Solid Edge part; units mm, degrees
sketch "Sketch1" plane through (0, 0, 0) normal (0, 0, 1) x (1, 0, 0)
  line L0 (6.35, 0) -> (6.35, 76.2)
  line L1 (6.35, 76.2) -> (22.225, 76.2)
  line L2 (22.225, 53.975) -> (22.225, 76.2)
  line L3 (22.225, 53.975) -> (98.425, 53.975)
  line L4 (98.425, 76.2) -> (98.425, 53.975)
  line L5 (98.425, 76.2) -> (114.3, 76.2)
  line L6 (114.3, 76.2) -> (114.3, 0)
  line L7 (114.3, 0) -> (98.425, 0)
  line L8 (98.425, 22.225) -> (98.425, 0)
  line L9 (98.425, 22.225) -> (22.225, 22.225)
  line L10 (22.225, 0) -> (22.225, 22.225)
  line L11 (22.225, 0) -> (6.35, 0)
  dimension "D1" = 6.35
  dimension "D2" = 22.225
  dimension "D3" = 6.35
extrude "Protrusion1" add sketch "Sketch1" along normal blind 12.7
hole "Hole_1" at (14.2875, 0, 6.35) direction (0, 1, 0) diameter 6.35 end through all
hole "Hole1" at (106.3625, 0, 6.35) direction (0, 1, 0) diameter 6.35 end through all
sketch "Sketch2" plane through (63.5, 38.1, 12.7) normal (0, 0, 1) x (1, 0, 0)
  line L0 (28.575, -9.525) -> (-34.925, -9.525)
  line L1 (-34.925, 9.525) -> (28.575, 9.525)
  arc A0 (-34.925, -9.525) -> (-34.925, 9.525) centre (-34.925, 0) cw
  arc A1 (28.575, 9.525) -> (28.575, -9.525) centre (28.575, 0) cw
extrude "Cutout1" cut sketch "Sketch2" against normal through all
fillet "Round_1" radius 12.7 4 edges at (22.225, 22.225, 6.35) (22.225, 53.975, 6.35) (98.425, 53.975, 6.35) (98.425, 22.225, 6.35)
sketch "Sketch3" plane through (60.325, 38.1, 12.7) normal (0, 0, 1) x (1, 0, 0)
  line L0 (-63.5, 38.1) -> (-63.5, -38.1)
  line L1 (-63.5, -38.1) -> (-50.8, -38.1)
  line L2 (-50.8, -38.1) -> (-50.8, 38.1)
  line L3 (-50.8, 38.1) -> (-63.5, 38.1)
  dimension "D1" = 63.5
extrude "ExtrudedProtrusion_2" add sketch "Sketch3" against normal blind 12.7
sketch "Sketch4" plane through (58.7375, 38.1, 12.7) normal (0, 0, 1) x (1, 0, 0)
  line L0 (-66.8536, -38.1) -> (-66.8536, -28.575)
  line L1 (-66.8536, -28.575) -> (-36.5125, -28.575)
  line L2 (-36.5125, -28.575) -> (-36.5125, -38.1)
  line L3 (-36.5125, -38.1) -> (-66.8536, -38.1)
  line L4 (-65.7913, 38.1) -> (-36.5125, 38.1)
  line L5 (-36.5125, 38.1) -> (-36.5125, 28.575)
  line L6 (-36.5125, 28.575) -> (-65.7913, 28.575)
  line L7 (-65.7913, 28.575) -> (-65.7913, 38.1)
  dimension "D1" = 65.7913
  dimension "D2" = 66.8536
extrude "Cutout2" cut sketch "Sketch4" against normal through all
fillet "Round_2" radius 3.175 8 edges at (98.425, 76.2, 6.35) (114.3, 76.2, 6.35) (114.3, 0, 6.35) (98.425, 0, 6.35) (22.225, 9.525, 6.35) (22.225, 66.675, 6.35) (-3.175, 66.675, 6.35) (-3.175, 9.525, 6.35)
sketch "Sketch5" plane through (55.5625, 38.1, 0) normal (0, 0, -1) x (0, 1, 0)
  line L0 (-38.1, -58.7375) -> (-38.1, -52.3875)
  line L1 (-38.1, -52.3875) -> (38.1, -52.3875)
  line L2 (38.1, -52.3875) -> (38.1, -58.7375)
  line L3 (38.1, -58.7375) -> (-38.1, -58.7375)
extrude "Cutout3" cut sketch "Sketch5" against normal through all
hole "Hole_11" at (3.175, 15.875, 6.35) direction (1, 0, 0) diameter 3.9675 end up to next
hole "Hole2" at (3.175, 60.325, 6.35) direction (1, 0, 0) diameter 3.9675 end up to next
properties part number "SR-03" material "Polyethylene, low density"
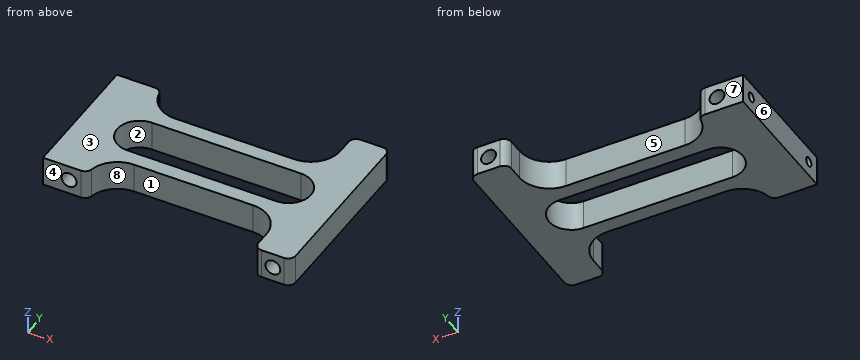
Input: part model. Units: mm. Frame: model coordinates. Face numbers are marked on the shaded views. A direction names the side the tool comes from. Round coordinates to 2 decimals unless told otherwise and drop trailing zeros. Write each loop counter-clockwise with the first axis right and the second up, starting at its lowest first coordinate (ties: lowest second). Pieces come first, ordered by that corner, then holes. Notation, with made-up numbers: M 0.25,-13.5 L 28.25,-13.5 A29 cw 28.25,18.5 Z; hole C 13,49.5 d1. An arc over 180 degrees is marked long. Write each question's results on one line, items separated by ' | '.
Q1. Line query: line 1 along Y through (x, z) = (7.75, 6.35) (3 decimals); line 2 along X through (y, z) = (50.5, 6.35) (1 decimal); line 3 along Y through (x, z) = (60, 2.5) (3 decimals). Output: solid intervals per line, ascending.
Results:
line 1: y = 9.525 to 13.891, 17.859 to 58.341, 62.309 to 66.675 | line 2: x = 3.2 to 11.1, 17.5 to 103.2, 109.5 to 114.3 | line 3: y = 22.225 to 28.575, 47.625 to 53.975
Q2. Draft query along X for the marked faces 6, 7 and 8. Return one class per face: released by +X, released by -X, zero draft, split by the parting line, or undercut.
Results:
face 6: released by -X | face 7: zero draft | face 8: undercut
Q3. Pin query (flat end, axial travel): P1, Ø1.5, axis at x = 47, z = 2, coming from the +Y side (3 decimals); P2, Ø6.5, axis at x = 65, z = 8.5, coming from the -Y side (3 decimals). Return the tip coordinate at first contact, or that it passes through.
Results:
P1: stops at y = 53.975 | P2: stops at y = 22.225
Q4. Section query A-A (y = 38.1). State how many separate pieces and enclosed holes the cut face has, and give its area (3 significant figures).
Results:
separate pieces: 2 | enclosed holes: 2 | area: 300 mm^2
Q5. Section query B-B (x = 75.5). Return loops of the section in (y, z) (3 decimals).
Results:
outline: M 22.225,0 L 28.575,0 L 28.575,12.7 L 22.225,12.7 Z; M 47.625,0 L 53.975,0 L 53.975,12.7 L 47.625,12.7 Z
Q6. Access query for the marked faces 1, 2, 3, 4 and 5. Directions: +Z, -Z, +X, -X, +Y, -Y. A direction counts if a zero-diameter tool reaches every point of the face in a straight line with its end or side. Return the directions, or none.
Results:
face 1: +Z, -Z, -Y | face 2: +Z, -Z | face 3: +Z, +X, -X, +Y, -Y | face 4: +Z, -Z, -X, -Y | face 5: +Z, -Z, +Y
